from build123d import *

# Parameters (mm, degrees)
SKETCH2_R           = 1.5
SKETCH2_R_2         = 4
BOSS_EXTRUDE1_DEPTH = 1.5
SKETCH6_R           = 1.5
CUT_EXTRUDE1_DEPTH  = 1.5
SKETCH7_R           = 1.5
CUT_EXTRUDE2_DEPTH  = 1.5


with BuildPart() as part:
    # Sketch2 → Boss-Extrude1 (new body)
    with BuildSketch(Plane(origin=(0, 0, 0), x_dir=(1, 0, 0), z_dir=(0, 1, 0))):
        with BuildLine():
            Line((0, -46.879161521), (0, -70.761127532))
            Line((0, -70.761127532), (15, -70.761127532))
            Line((15, -70.761127532), (23.677632731, -60.41952755))
            Line((23.677632731, -60.41952755), (129.929473623, -88.889622511))
            ThreePointArc((129.929473623, -88.889622511), (157.136079306, -83.55030532), (134.097880355, -68.124706791))
            Line((134.097880355, -68.124706791), (23.863280614, -38.592955603))
            Line((23.863280614, -38.592955603), (7.070663707, -26.834638658))
            Line((7.070663707, -26.834638658), (0, -35.261127532))
            Line((0, -35.261127532), (0, -44.643093543))
            ThreePointArc((0, -44.643093543), (0.5, -45.761127532), (0, -46.879161521))
        make_face()
        with Locations(Location((8, -40.761127532, 0), (0, 0, 90))):
            Circle(SKETCH2_R, mode=Mode.SUBTRACT)
        with Locations(Location((14, -50.761127532, 0), (0, 0, 90))):
            Circle(SKETCH2_R, mode=Mode.SUBTRACT)
        with Locations(Location((8, -60.761127532, 0), (0, 0, 90))):
            Circle(SKETCH2_R, mode=Mode.SUBTRACT)
        with Locations(Location((142.429473623, -80.598060535, 0), (0, 0, 90))):
            Circle(SKETCH2_R_2, mode=Mode.SUBTRACT)
        with BuildLine():
            Line((143.929473623, -73.498060535), (143.929473623, -68.998060535))
            ThreePointArc((143.929473623, -68.998060535), (142.429473623, -67.498060535), (140.929473623, -68.998060535))
            Line((140.929473623, -68.998060535), (140.929473623, -73.498060535))
            ThreePointArc((140.929473623, -73.498060535), (142.429473623, -74.998060535), (143.929473623, -73.498060535))
        make_face(mode=Mode.SUBTRACT)
        with BuildLine():
            Line((149.529473623, -82.098060535), (154.029473623, -82.098060535))
            ThreePointArc((154.029473623, -82.098060535), (155.529473623, -80.598060535), (154.029473623, -79.098060535))
            Line((154.029473623, -79.098060535), (149.529473623, -79.098060535))
            ThreePointArc((149.529473623, -79.098060535), (148.029473623, -80.598060535), (149.529473623, -82.098060535))
        make_face(mode=Mode.SUBTRACT)
        with BuildLine():
            Line((140.929473623, -87.698060535), (140.929473623, -92.198060535))
            ThreePointArc((140.929473623, -92.198060535), (142.429473623, -93.698060535), (143.929473623, -92.198060535))
            Line((143.929473623, -92.198060535), (143.929473623, -87.698060535))
            ThreePointArc((143.929473623, -87.698060535), (142.429473623, -86.198060535), (140.929473623, -87.698060535))
        make_face(mode=Mode.SUBTRACT)
        with BuildLine():
            Line((135.329473623, -79.098060535), (130.829473623, -79.098060535))
            ThreePointArc((130.829473623, -79.098060535), (129.329473623, -80.598060535), (130.829473623, -82.098060535))
            Line((130.829473623, -82.098060535), (135.329473623, -82.098060535))
            ThreePointArc((135.329473623, -82.098060535), (136.829473623, -80.598060535), (135.329473623, -79.098060535))
        make_face(mode=Mode.SUBTRACT)
    extrude(amount=BOSS_EXTRUDE1_DEPTH)

    # Sketch6 → Cut-Extrude1 (cut)
    with BuildSketch(Plane(origin=(0, 1.5, 0), x_dir=(1, 0, 0), z_dir=(0, 1, 0))):
        with Locations((31.86, -41.901127532)):
            Circle(SKETCH6_R)
    extrude(amount=-CUT_EXTRUDE1_DEPTH, mode=Mode.SUBTRACT)

    # Sketch7 → Cut-Extrude2 (cut)
    with BuildSketch(Plane(origin=(0, 1.5, 0), x_dir=(1, 0, 0), z_dir=(0, 1, 0))):
        with Locations(Location((74.014122572, -62.269648862, 0), (0, 0, 270))):
            Circle(SKETCH7_R)
        with Locations(Location((104.014122572, -70.306622169, 0), (0, 0, 270))):
            Circle(SKETCH7_R)
    extrude(amount=-CUT_EXTRUDE2_DEPTH, mode=Mode.SUBTRACT)


solid = part.part
Design review of the part built by this model. Coordinates are the model's own, in mm. A direction names the side the tool comes from. Give positions to 0.01 mm unless a question says otherwise; leave off trailing zeros. Loops run counter-clockwise (first coordinate to the right, second up) from the corner with the lowest first, then second, coordinate; pieces in that order, holes last. Notation, with made-up numbers: (40, 9.25) - (49, 9.25) arc R20 cw to (49, 35.25) - close; hole circle Ø1 at (27.25, 0.5). An arc over 180 degrees is marked (long way). Use CSV: the item, a comma, the result in double quotes. Start each with the question number.
1. Draft analysis for pull direction X (two halves, no side actions). For faces 1 (the flat face through (15.585, 0.74, 32.796)), 2 (the cylindrical face through (139.057, 0.74, 78.448)), 3 (the cylindrical face through (104.08, 0.76, 68.81)), 4 (the flat face through (78, 0, 61)), state which applies: released by +X, released by -X, zero draft, split by the parting line, or undercut.
2. Wall thickness on L1, parallel to Z at x = 14, y = 0.65; L2, parallel to Z at x = 79, y = 1.3; L3, parallel to Z at x = 136.5, y = 0.25: over which ranges is each line inside the solid? List them lowest first.
3. Insertion check: P1, Ø0.8, axis at x = 11, y = 0.5, coming from the +Z side. The pin has a flat end and moves straight along its axis. Give the tip position at first contact, or say it passes through.
4. Add section A-A (y = 0.5). Count the separate pieces of the cut face and the enclosed holes in it, plus the area to 3 significant figures.
5. Machinability: for faces 5 (the flat face through (76.06, 0.74, 74.455)), 6 (the flat face through (3.585, 0.74, 30.989)), which of the approach directions +Z, -Z, +X, -X, +Y, -Y give a long, thin tool a straight path to every point of the face, cutting with its end or side? Answer none if there is none.
6. Add section C-C (z = 57). State the section outline as (x, y) points, plus the area to 3 significant figures.
7. Add section B-B (x = 43.5). State the section outline as (y, z) points.
Results found:
1,face 1,"released by +X"
1,face 2,"undercut"
1,face 3,"undercut"
1,face 4,"zero draft"
2,L1,"z = 31.69 to 49.26, 52.26 to 70.76"
2,L2,"z = 53.36 to 75.24"
2,L3,"z = 66.82 to 79.66, 81.54 to 94.38"
3,P1,"stops at z = 70.76"
4,separate pieces,"1"
4,enclosed holes,"10"
4,area,"3,710 mm²"
5,face 5,"+Z, +Y, -Y"
5,face 6,"-Z, -X, +Y, -Y"
6,outline,"(0, 0) - (92.57, 0) - (92.57, 1.5) - (0, 1.5) - close"
6,area,"139 mm²"
7,outline,"(0, 43.85) - (1.5, 43.85) - (1.5, 65.73) - (0, 65.73) - close"
